For this review, take the finished solid that the model builds, in its own axes (mm). Face numbers are marked on the shaded views. A direction names the side the tool comes from. Round coordinates to 2 decimals unless told otherwise and drop trailing zeros. Loops run counter-clockwise (first coordinate to the right, second up) from the corner with the lowest first, then second, coordinate; pieces in that order, holes last. Notation, with made-up numbers: M 53,-7 L 64,-7 A15 ccw 64,1 Z; hole C 32,9 d10. An arc over 180 degrees is marked long. Write item = value, one per line. Start each with the question number.
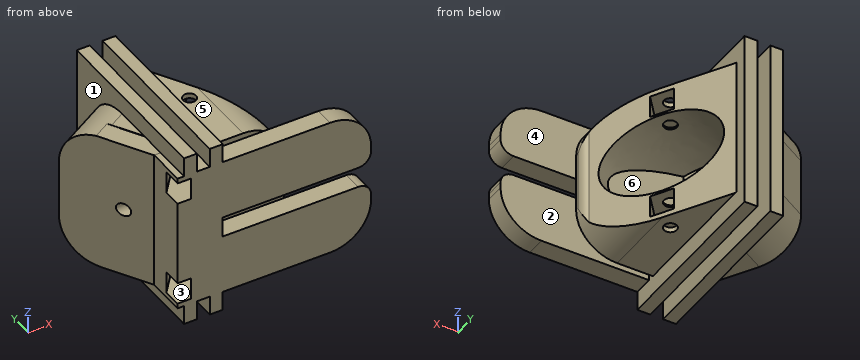
```python
from build123d import *

# Parameters (mm, degrees)
SKETCH2_W           = 21.7
SKETCH2_H           = 25.05
SKETCH2_RX          = 9.525
SKETCH2_RY          = 6.35
BOSS_EXTRUDE1_DEPTH = 12.7
SKETCH3_W           = 21.660653916
SKETCH3_H           = 25.05
BOSS_EXTRUDE2_DEPTH = 3
SKETCH5_W           = 18.892037138
SKETCH5_H           = 21.7
BOSS_EXTRUDE3_DEPTH = 2
SKETCH6_W           = 30
SKETCH6_H           = 21.7
BOSS_EXTRUDE4_DEPTH = 4
SKETCH7_W           = 21.7
SKETCH7_H           = 1
SKETCH7_W_2         = 3.175
SKETCH7_H_2         = 3
CUT_EXTRUDE2_DEPTH  = 23
SKETCH7_3_W         = 21.7
SKETCH7_3_H         = 7.272473706
CUT_EXTRUDE3_DEPTH  = 44.803879418
SKETCH11_R          = 1
CUT_EXTRUDE8_DEPTH  = 33.487034031
CUT_EXTRUDE4_REACH  = 47.088
SKETCH9_R           = 1
SKETCH15_W          = 3.4
SKETCH15_H          = 3.4
CUT_EXTRUDE9_DEPTH  = 28.443249332
BOSS_EXTRUDE5_DEPTH = 2
BOSS_EXTRUDE6_DEPTH = 2
FILLET5_R           = 6.35
FILLET6_R           = 2
FILLET7_R           = 2
SKETCH19_W          = 2
SKETCH19_H          = 4
CUT_EXTRUDE10_DEPTH = 48.148292291


with BuildPart() as part:
    # Sketch2 → Boss-Extrude1 (new body)
    with BuildSketch(Plane(origin=(16.497783942, 9.525, 0), x_dir=(0, 0, -1), z_dir=(0.8660254037844379, 0.5000000000000013, 0))):
        Rectangle(SKETCH2_W, SKETCH2_H)
        with Locations(Location((0, 0), (0, 0, 90))):
            Ellipse(SKETCH2_RX, SKETCH2_RY, mode=Mode.SUBTRACT)
    extrude(amount=-BOSS_EXTRUDE1_DEPTH)

    # Sketch3 → Boss-Extrude2 (add)
    with BuildSketch(Plane(origin=(5.499261314, 3.175, 0), x_dir=(0, 0, 1), z_dir=(-0.8660254037844379, -0.5000000000000014, 0))):
        with Locations((-0.019673042, 0)):
            Rectangle(SKETCH3_W, SKETCH3_H)
    extrude(amount=BOSS_EXTRUDE2_DEPTH)

    # Sketch5 → Boss-Extrude3 (add)
    with BuildSketch(Plane(origin=(0, 0, 0), x_dir=(-1, 0, 0), z_dir=(0, 1, 0))):
        with Locations((-13.314265373, 0)):
            Rectangle(SKETCH5_W, SKETCH5_H)
    extrude(amount=-BOSS_EXTRUDE3_DEPTH)

    # Sketch6 → Boss-Extrude4 (add)
    with BuildSketch(Plane.XZ.offset(2)):
        with Locations((18.868246804, 0)):
            Rectangle(SKETCH6_W, SKETCH6_H)
    extrude(amount=BOSS_EXTRUDE4_DEPTH)

    # Sketch7 → Cut-Extrude2 (cut)
    with BuildSketch(Plane(origin=(33.868246804, 0, 0), x_dir=(0, 0, -1), z_dir=(1, 0, 0))):
        with Locations((0, -2.5)):
            Rectangle(SKETCH7_W, SKETCH7_H)
        with Locations((0, -4.5)):
            Rectangle(SKETCH7_W_2, SKETCH7_H_2)
    extrude(amount=-CUT_EXTRUDE2_DEPTH, mode=Mode.SUBTRACT)

    # Sketch7<3> → Cut-Extrude3 (cut, through all)
    with BuildSketch(Plane(origin=(33.868246804, 0, 0), x_dir=(0, 0, -1), z_dir=(1, 0, 0))):
        with Locations((0, -9.636236853)):
            Rectangle(SKETCH7_3_W, SKETCH7_3_H)
    extrude(amount=-CUT_EXTRUDE3_DEPTH, mode=Mode.SUBTRACT)

    # Sketch11 → Cut-Extrude8 (cut, through all)
    with BuildSketch(Plane(origin=(19.672783942, 0.194872981, 0), x_dir=(0, 0, -1), z_dir=(-1, 0, 0))):
        with Locations(Location((0, -3.830865705, 0), (0, 0, 90))):
            Circle(SKETCH11_R)
    extrude(amount=CUT_EXTRUDE8_DEPTH, mode=Mode.SUBTRACT)

    # Sketch9 → Cut-Extrude4 (cut, up to next)
    with BuildSketch(Plane(origin=(0, 0, -10.85), x_dir=(-1, 0, 0), z_dir=(0, 0, -1)), mode=Mode.PRIVATE) as cut_extrude4_sk1:
        with Locations((-14.332720433, 8.275)):
            Circle(SKETCH9_R)
    cut_extrude4_tool1 = extrude(cut_extrude4_sk1.sketch, amount=-CUT_EXTRUDE4_REACH, mode=Mode.PRIVATE) & part.part
    cut_extrude4 = cut_extrude4_tool1.solids().sort_by_distance((14.33272, 8.275, -10.85))[0]
    add(cut_extrude4, mode=Mode.SUBTRACT)

    # Sketch15 → Cut-Extrude9 (cut, symmetric)
    with BuildSketch(Plane(origin=(16.497783942, 9.525, 0), x_dir=(0.7757354378747654, -0.6310582623064579, 0), z_dir=(0.6310582623064579, 0.7757354378747654, 0))):
        with Locations((-0.1, -8.35)):
            Rectangle(SKETCH15_W, SKETCH15_H)
    cut_extrude9 = extrude(amount=CUT_EXTRUDE9_DEPTH, both=True, mode=Mode.SUBTRACT)

    # Sketch16 → Boss-Extrude5 (add)
    with BuildSketch(Plane(origin=(8.868246804, 0, 0), x_dir=(0, 0, -1), z_dir=(1, 0, 0))):
        Polygon((-10.85, -6), (-10.85, 19.582708922), (0, 19.582708922), (0, 21.582708922), (-13.85, 21.582708922), (-13.85, -6), align=None)
    boss_extrude5 = extrude(amount=BOSS_EXTRUDE5_DEPTH)

    # Sketch18 → Boss-Extrude6 (add)
    with BuildSketch(Plane.ZY.offset(-6.868246804)):
        Polygon((10.85, -6), (13.85, -6), (13.85, 21.582708922), (0, 21.582708922), (0, 14.582708922), (10.85, 14.582708922), align=None)
    boss_extrude6 = extrude(amount=BOSS_EXTRUDE6_DEPTH)

    # Mirror1: Cut-Extrude4, Cut-Extrude9, Boss-Extrude5, Boss-Extrude6 across plane
    add(cut_extrude4.mirror(Plane.XY), mode=Mode.SUBTRACT)
    add(cut_extrude9.mirror(Plane.XY), mode=Mode.SUBTRACT)
    add(boss_extrude5.mirror(Plane.XY))
    add(boss_extrude6.mirror(Plane.XY))

    # Fillet5
    fillet5_edges = [part.edges().sort_by_distance(p)[0] for p in [
        (22.760283942, -1, 10.85),
        (22.760283942, -1, -10.85),
        (0.753465953, 14.897638014, -10.85),
        (2.052504059, 15.647638014, 10.85),
        (33.868246804, -4.5, -10.85),
        (33.868246804, -4.5, 10.85),
    ]]
    fillet(fillet5_edges, radius=FILLET5_R)

    # Fillet6
    fillet6_edges = [part.edges().sort_by_distance(p)[0] for p in [
        (33.868246804, -4.5, 1.5875),
        (33.868246804, -4.5, -1.5875),
    ]]
    fillet(fillet6_edges, radius=FILLET6_R)

    # Fillet7
    # the kernel refuses this fillet: 2 mm, written as the material it takes off along each edge
    with BuildSketch(Plane(origin=(22.760283942, 0, 8.429393602), x_dir=(0, -1, 0), z_dir=(0, 0, -1))) as fillet7_piece_1:
        with BuildLine():
            CenterArc((1.571757441, 2), FILLET7_R, 218.197977663, 51.802022337)
            Line((0, 0.763238686), (-0.031435149, 0.73850346))
            ThreePointArc((-0.031435149, 0.73850346), (-0.04, 0.381619343), (-0.04, 0))
            Line((-0.04, 0), (0, -0.04))
            Line((0, -0.04), (1.571757441, -0.04))
            Line((1.571757441, -0.04), (1.571757441, 0))
        make_face()
    extrude(amount=16.858787203, mode=Mode.SUBTRACT)

    # Sketch19 → Cut-Extrude10 (cut, through all)
    with BuildSketch(Plane.XY.offset(10.85)):
        with Locations((7.868246804, 19.582708922)):
            Rectangle(SKETCH19_W, SKETCH19_H)
    extrude(amount=-CUT_EXTRUDE10_DEPTH, mode=Mode.SUBTRACT)


solid = part.part
```
(1) Add section C-C on z = -8. Write out the cut boundary in (x, y) (3 decimals).
(2) Add section A-A on x = 27. Write out the cut boundary in (y, z), and give its area (3 significant figures).
(3) Draft analysis for pull direction X (two halves, no side actions). For the marked faces 1, 2 and 3, state which applies: +X half, -X half, draft (parallel to the pull), parting line (faces both ways), or undercut.
(4) Tool access review of the marked faces 4, 5 and 6: name each direction out of +Z, -Z, +X, -X, +Y, -Y from which nothing blocks a thin tool from reaching the whole face with its end or side.
(5) Add section B-B on y = 20.25. Write out the cut boundary in (x, z), and give its area (3 significant figures).
(6) For pin 1 Ø10 at (y, z) = (3, -5) entering from +X; pin 2 Ø14 at (y, z) = (1, 0) entering from -X; pin 3 Ø2.5 at (x, y) = (24, -4.5) entering from -Z, all flat-tipped, find the tip position at first contact; note any pin that passes through.
(7) Wall thickness on L1, parallel to X at y = -3, z = -12; L2, parallel to Y at x = 3.3, z = 0; L3, parallel to X at y = -0.25, z = -7: over which ranges is each line inside the solid? List them lowest first.
(8) Add section D-D on y = -0.5. Count the separate pieces of the cut face and the enclosed holes in it, and give its area (3 significant figures).
Answer sheet:
q1.outline = M -2.835,11.611 L 3.868,0 L 3.868,-3.148 L 13.365,8.526 A1 cw 13.89,9.172 L 15.535,11.193 L 10.691,19.583 L 10.868,19.583 L 10.868,21.583 L 8.868,21.583 L 8.868,17.583 L 6.868,17.583 L 6.868,21.583 L 4.868,21.583 L 4.868,16.059 Z; M 5.931,-6 L 32.817,-6 L 32.817,-3 L 10.868,-3 L 10.868,-2 L 21.709,-2 L 21.709,0.5 L 17.354,8.042 Z
q2.outline = M -6,-10.85 L -3,-10.85 L -3,-1.59 L -6,-1.59 Z; M -6,1.59 L -3,1.59 L -3,10.85 L -6,10.85 Z
q2.area = 55.6 mm²
q3.face_1 = -X half
q3.face_2 = draft
q3.face_3 = undercut
q4.face_4 = +Z, -Z, +X
q4.face_5 = +Z, +X, +Y, -Y
q4.face_6 = none
q5.outline = M 4.87,-13.85 L 6.87,-13.85 L 6.87,13.85 L 4.87,13.85 Z; M 8.87,-13.85 L 10.87,-13.85 L 10.87,13.85 L 8.87,13.85 Z
q5.area = 111 mm²
q6.pin_1 = 22.76
q6.pin_2 = -0.75
q6.pin_3 = -10.85
q7.L1 = 4.87 to 6.87, 8.87 to 10.87
q7.L2 = 0.98 to 3.03, 5.03 to 6.98, 12.9 to 16.37
q7.L3 = 3.87 to 6.23, 10.61 to 22.25
q8.separate_pieces = 1
q8.enclosed_holes = 2
q8.area = 383 mm²
